Geometry check sheet. Reference: drawing and pictorial views, mm from the part's lowest x, y, z. A direction names the side the tool comes from. Give positions to 0.01 mm unless a question says otherwise; leave off trailing zeros. Loops run counter-clockwise (first coordinate to the right, second up) from the corner with the lowest first, then second, coordinate; pieces in that order, holes last. Notation, with made-up numbers: (-22, 32.5) - (-8, 32.5) arc R22 ccw to (-8, 51.5) - close; hole circle Ø6 at (32.25, 57.25). An arc over 180 degrees is marked (long way). Use CSV: the item, a comma, the result in double quotes.
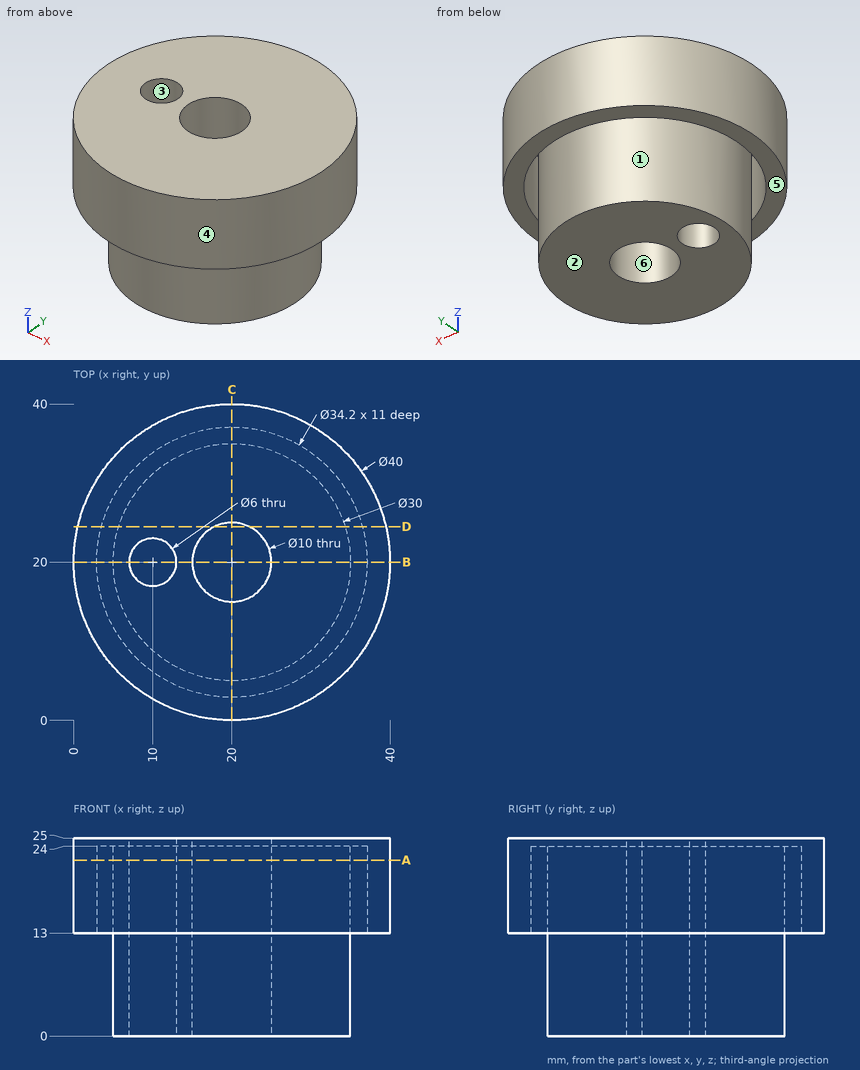
1. Release check for a two-part mould opening along Y. For the marked faces 3, 4, 5 and 6 record: released by +Y, released by -Y, zero draft, split by the parting line, or undercut.
Completed:
face 3,"undercut"
face 4,"split by the parting line"
face 5,"zero draft"
face 6,"undercut"
2. Sectioned sample at D-D, the plane y = 24.5. Record the boundary of the cut face in (x, z).
Completed:
outline,"(0.51, 13) - (3.5, 13) - (3.5, 24) - (5.69, 24) - (5.69, 0) - (17.82, 0) - (17.82, 25) - (0.51, 25) - close; (22.18, 0) - (34.31, 0) - (34.31, 24) - (36.5, 24) - (36.5, 13) - (39.49, 13) - (39.49, 25) - (22.18, 25) - close"
3. Go/stop test with flat-tipped pins: pin 1 Ø1.5 at (x, z) = (30, 9) entering from +Y; pin 2 Ø1 at (y, z) = (18, 13.5) entering from -X; pin 3 Ø3 at (y, z) = (14.5, 19) entering from -X. Record where each tip stops, or that it passes through.
Completed:
pin 1,"stops at y = 31.81"
pin 2,"stops at x = 0.06"
pin 3,"stops at x = 0.4"
4. Set-up check for the marked faces 1 and 2: record each of +Z, -Z, +X, -X, +Y, -Y from which the full face is reachable in a straight line by a thin tool's end or side.
Completed:
face 1,"-Z"
face 2,"-Z, +X, -X, +Y, -Y"
5. Scan lines: line 1 along Y through (x, z) = (20, 15.5); line 2 along Y through (x, z) = (20, 9.25); line 3 along X through (y, z) = (28.5, 16.25). Record each from-to range of solid material in increasing order.
Completed:
line 1,"y = 0 to 2.9, 5 to 15, 25 to 35, 37.1 to 40"
line 2,"y = 5 to 15, 25 to 35"
line 3,"x = 1.9 to 5.16, 7.64 to 32.36, 34.84 to 38.1"
6. Sectioned sample at C-C, the plane x = 20. Record the boundary of the cut face in (y, z).
Completed:
outline,"(0, 13) - (2.9, 13) - (2.9, 24) - (5, 24) - (5, 0) - (15, 0) - (15, 25) - (0, 25) - close; (25, 0) - (35, 0) - (35, 24) - (37.1, 24) - (37.1, 13) - (40, 13) - (40, 25) - (25, 25) - close"
7. Sectioned sample at A-A, the plane z = 22.25. Record the boundary of the cut face in (x, y).
Completed:
outline,"circle Ø40 at (20, 20); circle Ø30 at (20, 20); hole circle Ø34.2 at (20, 20); hole circle Ø6 at (10, 20); hole circle Ø10 at (20, 20)"
8. Sectioned sample at B-B, the plane y = 20. Record the boundary of the cut face in (x, z).
Completed:
outline,"(0, 13) - (2.9, 13) - (2.9, 24) - (5, 24) - (5, 0) - (7, 0) - (7, 25) - (0, 25) - close; (13, 0) - (15, 0) - (15, 25) - (13, 25) - close; (25, 0) - (35, 0) - (35, 24) - (37.1, 24) - (37.1, 13) - (40, 13) - (40, 25) - (25, 25) - close"
